Source: CAD feature listing. Evaluate the final solid. Frame: model axes, mm. Coordinates: 2 decimals unless noted, no trailing zeros. Write each loop counter-clockwise with the first axis right and the second up, starting at its lowest first coordinate (ties: lowest second). Pieces come first, ordered by that corner, then holes. Notation, with made-up numbers: M 39,85 L 81,85 A25 ccw 81,115 Z; hole C 13,45 d1. An arc over 180 degrees is marked long. Answer as CSV lines item,"result". Start each with the question number.
1. Contact query for flat-ended pins moving along their axis: pin 1 Ø4 at (x, z) = (-3.5, -10.5) entering from +Y; pin 2 Ø4 at (x, z) = (-12.5, 9.5) entering from -Y; pin 3 Ø8 at (x, y) = (4, -15.5) entering from +Z. Output: stop coordinate, or through.
2. Section A-A on z = 10.5. Return the cut outline in (x, y).
3. Line query: probe 1 along Z at (x, y) = (0, -10.25); probe 2 along Z at (x, y) = (0, -4); probe 3 along X at (y, z) = (-8.5, 5). Output: solid intervals per line, ascending. Write a range as [from, to].
4. Section B-B on z = -3. Return the cut outline in (x, y), plus the area to 3 significant figures.
```python
from build123d import *

# Parameters (mm, degrees)
F3_DEPTH = 21.844
F4_R     = 9.652
F5_DEPTH = 21.844


with BuildPart() as f1:
    # F0 (on Front) → F1 (revolve)
    with BuildSketch(Plane.XZ):
        with BuildLine():
            Line((-21.59, -24.892), (0, -24.892))
            Line((0, -24.892), (0, 0))
            Line((0, 0), (0, 42.164))
            ThreePointArc((0, 42.164), (-12.216408, 40.104491), (-21.59, 32.004))
            Line((-21.59, 32.004), (-21.59, 19.304))
            Line((-21.59, 19.304), (-21.59, 0))
            Line((-21.59, 0), (-21.59, -24.892))
        make_face()
    revolve(axis=Axis((0, 0, 8.636), (0, 0, -1)))

    # F2 (on Front) → F3 (cut)
    with BuildSketch(Plane.XZ):
        with BuildLine():
            ThreePointArc((0, 19.304), (-9.652, 9.652), (0, 0))
            Line((0, 0), (0, 19.304))
        make_face()
        with BuildLine():
            Line((0, 19.304), (0, 0))
            ThreePointArc((0, 0), (6.824995, 2.827005), (9.652, 9.652))
            ThreePointArc((9.652, 9.652), (6.824995, 16.476995), (0, 19.304))
        make_face()
    extrude(amount=-F3_DEPTH, mode=Mode.SUBTRACT)

    # F4 (on Front) → F5 (cut)
    with BuildSketch(Plane.XZ):
        with Locations((0, 9.652)):
            Circle(F4_R)
    extrude(amount=F5_DEPTH, mode=Mode.SUBTRACT)


solid = f1.part
```
Values:
1,pin 1,"y = 21.54"
1,pin 2,"y = -18.86"
1,pin 3,"z = 40.2"
2,outline,"M -9.61,-19.33 L -9.61,19.33 A21.59 ccw Z; M 9.61,-19.33 A21.59 ccw 9.61,19.33 Z"
3,probe 1,"[-24.89, 0], [19.3, 40.92]"
3,probe 2,"[-24.89, 0], [19.3, 42.24]"
3,probe 3,"[-19.85, -8.46], [8.46, 19.85]"
4,outline,"C 0,0 d43.18"
4,area,"1,460 mm²"
